```python
from build123d import *

# Parameters (mm, degrees)
SKETCH_1_W          = 100
SKETCH_1_H          = 30
EXTRUDE_1_DEPTH     = 50
SKETCH_2_W          = 41
SKETCH_2_H          = 20
CUT_EXTRUDE_1_DEPTH = 37
SKETCH_3_W          = 7
SKETCH_3_H          = 19
CUT_EXTRUDE_2_DEPTH = 8
SKETCH_4_W          = 7
SKETCH_4_H          = 7
CUT_EXTRUDE_3_DEPTH = 29
SKETCH_5_W          = 48
SKETCH_5_H          = 7
CUT_EXTRUDE_4_DEPTH = 5
CUT_EXTRUDE_5_REACH = 80.063
SKETCH_6_W          = 5
SKETCH_6_H          = 7
CUT_EXTRUDE_6_REACH = 84.643
SKETCH_7_R          = 2.5


with BuildPart() as part:
    # 草圖1 → 填料-伸長1 (new body)
    with BuildSketch(Plane.XY):
        with Locations((13.030079174, 3.895348837)):
            Rectangle(SKETCH_1_W, SKETCH_1_H)
    extrude(amount=EXTRUDE_1_DEPTH)

    # 草圖2 → 除料-伸長1 (cut)
    with BuildSketch(Plane.XY.offset(50)):
        with Locations((3.530079174, 3.895348837)):
            Rectangle(SKETCH_2_W, SKETCH_2_H)
    extrude(amount=-CUT_EXTRUDE_1_DEPTH, mode=Mode.SUBTRACT)

    # 草圖3 → 除料-伸長2 (cut)
    with BuildSketch(Plane.XY.offset(50)):
        with Locations((27.530079174, 3.895348837)):
            Rectangle(SKETCH_3_W, SKETCH_3_H)
        with Locations((-20.469920826, 3.895348837)):
            Rectangle(SKETCH_3_W, SKETCH_3_H)
    extrude(amount=-CUT_EXTRUDE_2_DEPTH, mode=Mode.SUBTRACT)

    # 草圖4 → 除料-伸長3 (cut)
    with BuildSketch(Plane.XY.offset(42)):
        with Locations((-20.469920826, 3.895348837)):
            Rectangle(SKETCH_4_W, SKETCH_4_H)
    extrude(amount=-CUT_EXTRUDE_3_DEPTH, mode=Mode.SUBTRACT)

    # 草圖5 → 除料-伸長4 (cut)
    with BuildSketch(Plane.XY.offset(13)):
        with Locations((0.030079174, 3.895348837)):
            Rectangle(SKETCH_5_W, SKETCH_5_H)
    extrude(amount=-CUT_EXTRUDE_4_DEPTH, mode=Mode.SUBTRACT)

    # 草圖6 → 除料-伸長5 (cut, up to next)
    with BuildSketch(Plane.XY.offset(8), mode=Mode.PRIVATE) as cut_extrude_5_sk1:
        with Locations((21.530079174, 3.895348837)):
            Rectangle(SKETCH_6_W, SKETCH_6_H)
    cut_extrude_5_tool1 = extrude(cut_extrude_5_sk1.sketch, amount=-CUT_EXTRUDE_5_REACH, mode=Mode.PRIVATE) & part.part
    add(cut_extrude_5_tool1.solids().sort_by_distance((21.530079, 3.895349, 8))[0], mode=Mode.SUBTRACT)

    # 草圖7 → 除料-伸長6 (cut, up to next)
    with BuildSketch(Plane(origin=(0, 0, 0), x_dir=(-1, 0, 0), z_dir=(0, 0, -1)), mode=Mode.PRIVATE) as cut_extrude_6_sk1:
        with Locations((7.969920826, 3.895348837)):
            Circle(SKETCH_7_R)
    cut_extrude_6_tool1 = extrude(cut_extrude_6_sk1.sketch, amount=-CUT_EXTRUDE_6_REACH, mode=Mode.PRIVATE) & part.part
    add(cut_extrude_6_tool1.solids().sort_by_distance((-7.969921, 3.895349, 0))[0], mode=Mode.SUBTRACT)


solid = part.part
```
Geometry check sheet. Reference: the model listing, model coordinates, mm. A direction names the side the tool comes from. Round coordinates to 2 decimals unless told otherwise and drop trailing zeros. Loops run counter-clockwise (first coordinate to the right, second up) from the corner with the lowest first, then second, coordinate; pieces in that order, holes last. Notation, with made-up numbers: M -31,-31 L 2,-31 A28 ccw 2,-9 Z; hole C 83,82 d10. An arc over 180 degrees is marked long. Return JSON: item names as keys, results as strings. Group by question number.
(1) Go/stop test with flat-tipped pins: pin 1 (2 mm diameter, centred on x = 4.5, y = -1.5, fed in from +Z); pin 2 (1.8 mm diameter, centred on x = -20, y = 11.5, fed in from +Z); pin 3 (2 mm diameter, centred on x = -18.5, y = 13.5, fed in from -Z); pin 4 (6 mm diameter, centred on x = -7.97, y = 3.9, fed in from +Z). Record where each tip stops, or that it passes through.
(2) Section check D-D, the plane z = 45. Enter the section's corners in (x, y), and give its area (3 significant figures).
(3) Set-up check for faces 5 (the face through (63.03, 4, 25)), 6 (the face through (-21, -5.605, 46)): record each of +Z, -Z, +X, -X, +Y, -Y from which the full face is reachable in a straight line by a thin tool's end or side.
(4) Scan lines: line 1 along X through (y, z) = (3, 34); line 2 along Y through (x, z) = (13.5, 16); line 3 along Y through (x, z) = (-18, 35.5). Record each from-to range of solid material in increasing order. Write a range as [from, to].
(5) Section check C-C, the plane x = -7.5. Enter the section's corners in (y, z).
(6) Section check A-A, the plane z = 36.5. Enter the section's corners in (x, y), and give its area (3 significant figures).
(7) Mould release check, pull along X, two halves, no side actions. Record for faces 1 (the face through (23.4, 14.1, 50)), 2 (the face through (-36.97, 4, 25)), 3 (the face through (-21, -3, 42)), 4 (the face through (27, 13.395, 46)): pulls with the +X half, pulls with the -X half, needs draft (parallel to the pull), parting line crosses it, or undercut.
(8) Section check B-B, the plane x = 30. Enter the section's corners in (y, z), and give its area (3 significant figures).
Data:
{
 "1": {"pin 1": "z = 13", "pin 2": "z = 42", "pin 3": "z = 0", "pin 4": "z = 8"},
 "2": {"outline": "M -36.97,-11.1 L 63.03,-11.1 L 63.03,18.9 L -36.97,18.9 Z; hole M -23.97,-5.6 L -16.97,-5.6 L -16.97,-6.1 L 24.03,-6.1 L 24.03,-5.6 L 31.03,-5.6 L 31.03,13.4 L 24.03,13.4 L 24.03,13.9 L -16.97,13.9 L -16.97,13.4 L -23.97,13.4 Z", "area": "1,910 mm²"},
 "3": {"face 5": "+Z, -Z, +X, +Y, -Y", "face 6": "+Z"},
 "4": {"line 1": "[-36.97, -23.97], [24.03, 63.03]", "line 2": "[-11.1, -6.1], [13.9, 18.9]", "line 3": "[-11.1, 0.4], [7.4, 18.9]"},
 "5": {"outline": "M -11.1,0 L 1.44,0 L 1.44,8 L 0.4,8 L 0.4,13 L -6.1,13 L -6.1,50 L -11.1,50 Z; M 6.35,0 L 18.9,0 L 18.9,50 L 13.9,50 L 13.9,13 L 7.4,13 L 7.4,8 L 6.35,8 Z"},
 "6": {"outline": "M -36.97,-11.1 L 63.03,-11.1 L 63.03,18.9 L -36.97,18.9 Z; hole M -23.97,0.4 L -16.97,0.4 L -16.97,-6.1 L 24.03,-6.1 L 24.03,13.9 L -16.97,13.9 L -16.97,7.4 L -23.97,7.4 Z", "area": "2,130 mm²"},
 "7": {"face 1": "needs draft", "face 2": "pulls with the -X half", "face 3": "undercut", "face 4": "undercut"},
 "8": {"outline": "M -11.1,0 L 18.9,0 L 18.9,50 L 13.4,50 L 13.4,42 L -5.6,42 L -5.6,50 L -11.1,50 Z", "area": "1,350 mm²"}
}
